Build history of the part. All positions in model axes, mm. A direction names the side the tool comes from. Round coordinates to 2 decimals unless told otherwise and drop trailing zeros. Write each loop counter-clockwise with the first axis right and the second up, starting at its lowest first coordinate (ties: lowest second). Pieces come first, ordered by that corner, then holes.
Autodesk Inventor part; units mm, degrees
ref_plane "YZ Plane" through (0, 0, 0) normal (1, 0, 0) x (0, 1, 0)
ref_plane "XZ Plane" through (0, 0, 0) normal (0, 1, 0) x (-1, 0, 0)
ref_plane "XY Plane" through (0, 0, 0) normal (0, 0, 1) x (1, 0, 0)
sketch "Sketch1" plane through (0, 0, 0) normal (0, 0, 1) x (1, 0, 0)
  line L0 (-25, -15) -> (25, -15)
  line L1 (25, -15) -> (25, 15)
  line L2 (25, 15) -> (-25, 15) construction
  line L3 (-25, 15) -> (-25, -15)
  line L4 (-25, -15) -> (25, 15) construction
  line L5 (25, -15) -> (-25, 15) construction
  line L6 (-25, 15) -> (-30, 15)
  line L7 (-30, 15) -> (-30, -20)
  line L8 (-30, -20) -> (30, -20)
  line L9 (30, -20) -> (30, 15)
  line L10 (30, 15) -> (25, 15)
  point P0 (0, 0)
  dimension "d0" = 50
  dimension "d1" = 30
  dimension "d2" = 5
  dimension "d3" = 35
  dimension "d4" = 60
extrude "Extrusion1" add sketch "Sketch1" along normal blind 180
properties part number "track 1832"
1) Slice it at B-B (z = 158). Write the cut outline in (x, y), plus the area to 3 significant figures.
Results:
outline: (-30, -20) - (30, -20) - (30, 15) - (25, 15) - (25, -15) - (-25, -15) - (-25, 15) - (-30, 15) - close
area: 600 mm2
2) Mould opens along X. For faces 3 (the flat face through (-27, 15, 89)), 4 (the flat face through (-25, 0, 89)), 5 (the flat face through (-30, -2, 89)) say: released by +X, released by -X, zero draft, split by the parting line, or undercut.
Results:
face 3: zero draft
face 4: undercut
face 5: released by -X
3) Slice it at A-A (y = -3). Write the cut outline in (x, z).
Results:
outline: (-30, 0) - (-25, 0) - (-25, 180) - (-30, 180) - close; (25, 0) - (30, 0) - (30, 180) - (25, 180) - close
4) Pin check, flat tips, straight feed: pin 1 Ø10 at (x, z) = (-21, 87.5) entering from +Y; pin 2 Ø25 at (x, z) = (9, 73.5) entering from +Y. Stop position of each tip, or through.
Results:
pin 1: stops at y = 15
pin 2: stops at y = -15
5) Wall check: L1, parallel to X at y = 8.5, z = 105.5; L2, parallel to Y at x = -20, z = 165. Give the ranges that are in metal, low to high.
Results:
L1: x = -30 to -25, 25 to 30
L2: y = -20 to -15
6) Which spindle directions (+Z, -Z, +X, -X, +Y, -Y) get a long thin tool onto all of the face, cutting with end or side? Do faces 1 (the flat face through (28, 15, 89)), 2 (the flat face through (0, -15, 89)). Say none if no direction does.
Results:
face 1: +Z, -Z, +X, -X, +Y
face 2: +Z, -Z, +Y
7) Slice it at C-C (x = 4). Write the cut outline in (y, z), plus the area to 3 significant figures.
Results:
outline: (-20, 0) - (-15, 0) - (-15, 180) - (-20, 180) - close
area: 900 mm2
